from build123d import *

# Parameters (mm, degrees)
BOSS_EXTRUDE1_DEPTH        = 7.5
CUT_EXTRUDE1_DEPTH         = 1.5
F_3_1_3_1_DIAMETER_HOLE1_D = 3.1


with BuildPart() as part:
    # Sketch1 → Boss-Extrude1 (new body)
    with BuildSketch(Plane(origin=(0, 0, 0), x_dir=(1, 0, 0), z_dir=(0, 1, 0))):
        with BuildLine():
            Line((-219.119725045, 38.636719531), (-204.34760875, 36.031996866))
            ThreePointArc((-204.34760875, 36.031996866), (-207.5, 0), (-204.34760875, -36.031996866))
            Line((-204.34760875, -36.031996866), (-219.119725045, -38.636719531))
            ThreePointArc((-219.119725045, -38.636719531), (-222.5, 0), (-219.119725045, 38.636719531))
        make_face()
    extrude(amount=BOSS_EXTRUDE1_DEPTH)

    # Sketch2 → Cut-Extrude1 (cut)
    with BuildSketch(Plane(origin=(0, 7.5, 0), x_dir=(1, 0, 0), z_dir=(0, 1, 0))):
        with BuildLine():
            Line((-206.809628133, 36.46611731), (-216.657705663, 38.202599087))
            ThreePointArc((-216.657705663, 38.202599087), (-218.670303662, 24.151569236), (-219.772609758, 10))
            Line((-219.772609758, 10), (-209.761769634, 10))
            ThreePointArc((-209.761769634, 10), (-208.70564487, 23.279901188), (-206.809628133, 36.46611731))
        make_face()
        with BuildLine():
            Line((-209.761769634, -10), (-219.772609758, -10))
            ThreePointArc((-219.772609758, -10), (-218.670303662, -24.151569236), (-216.657705663, -38.202599087))
            Line((-216.657705663, -38.202599087), (-206.809628133, -36.46611731))
            ThreePointArc((-206.809628133, -36.46611731), (-208.70564487, -23.279901188), (-209.761769634, -10))
        make_face()
    extrude(amount=-CUT_EXTRUDE1_DEPTH, mode=Mode.SUBTRACT)

    # Ø3.1 (3.1) Diameter Hole1 (through all)
    with Locations(Plane(origin=(0, 0, 0), x_dir=(-1, 0, 0), z_dir=(0, -1, 0))):
        with Locations((214.18186009, -18.738484691), (214.18186009, 18.738484691)):
            Hole(F_3_1_3_1_DIAMETER_HOLE1_D / 2)


solid = part.part
Read the model definition and answer for the solid it produces. Units are mm, in the model's axes. A direction names the side the tool comes from. Round coordinates to 2 decimals unless told otherwise and drop trailing zeros. Order: outer loops, then holes, each group sorted by start corner. A loop starts at its lowest first (then second) coordinate and runs counter-clockwise, first axis right, second up.
1) For faces 5 (the face through (-208.726, 6.76, -23.095)), 6 (the face through (-208.685, 6.76, 23.465)), 7 (the face through (-215, 7, 10)), 8 (the face through (-207.5, 3.7, -0.5)), 9 (the face through (-212.75, 3.04, 19.33)), determine the directions among +Z, -Z, +X, -X, +Y, -Y from which every point of the face is accessible in a straight line to the end or side of a thin tool.
2) The part is cut by section B-B on y = 1. Write down the section's boundary in (x, z).
3) The part is cut by section C-C on x = -208.5. Write down the section's boundary in (y, z), plus the area to 3 significant figures.
4) Flat-ended cylindrical pins translate along their axes: pin 1 (2.5 mm diameter, centred on x = -214.18, z = 18.74, fed in from -Y); pin 2 (1 mm diameter, centred on y = 5, z = 12, fed in from -X); pin 3 (1.6 mm diameter, centred on x = -214, y = 7, fed in from -Z); pin 4 (2 mm diameter, centred on y = 3.5, z = -23.5, fed in from +X). Find the tip coordinate at first contact, or state that the pin passes through.
5) The mould has two halves that part along Z. Classify faces 1 (the face through (-218.692, 6.76, 23.954)), 2 (the face through (-222.5, 3.7, 0.5)), 3 (the face through (-215, 7.5, -1)), 4 (the face through (-211.63, 2.864, 37.316)): released by +Z, released by -Z, zero draft, split by the parting line, or undercut.
6) Straight lines are drawn through the part: L1, parallel to Z at x = -214, y = 3.25; L2, parallel to X at y = 3.25, z = 2; L3, parallel to Y at x = -209.5, z = -15. For each, find the intervals that lie inside material, in ascending order.
7) The part is cut by section D-D on y = 6.75. Write down the section's boundary in (x, z), plus the area to 3 significant figures.
8) The part is cut by section A-A on z = 18. Write down the section's boundary in (x, y).
Resolved:
1. face 5: -Z, +Y
1. face 6: +Z, +Y
1. face 7: +Y
1. face 8: +X, +Y, -Y
1. face 9: +Y, -Y
2. outline: (-219.12, -38.64) - (-204.35, -36.03) arc R207.5 cw to (-204.35, 36.03) - (-219.12, 38.64) arc R222.5 ccw to start; hole circle Ø3.1 at (-214.18, -18.74); hole circle Ø3.1 at (-214.18, 18.74)
3. outline: (0, -36.76) - (6, -36.76) - (6, -25.05) - (7.5, -25.05) - (7.5, 25.05) - (6, 25.05) - (6, 36.76) - (0, 36.76) - close
3. area: 516 mm2
4. pin 1: passes through
4. pin 2: stops at x = -222.2
4. pin 3: stops at z = -10
4. pin 4: stops at x = -206.05
5. face 1: undercut
5. face 2: split by the parting line
5. face 3: zero draft
5. face 4: released by +Z
6. L1: z = -37.73 to -20.28, -17.2 to 17.2, 20.28 to 37.73
6. L2: x = -222.49 to -207.49
6. L3: y = 0 to 6
7. outline: (-219.77, -10) - (-209.76, -10) arc R210 ccw to (-206.81, -36.47) - (-204.35, -36.03) arc R207.5 cw to (-204.35, 36.03) - (-206.81, 36.47) arc R210 ccw to (-209.76, 10) - (-219.77, 10) arc R220 cw to (-216.66, 38.2) - (-219.12, 38.64) arc R222.5 ccw to (-219.12, -38.64) - (-216.66, -38.2) arc R220 cw to start
7. area: 575 mm2
8. outline: (-221.77, 0) - (-215.54, 0) - (-215.54, 6) - (-219.26, 6) - (-219.26, 7.5) - (-221.77, 7.5) - close; (-212.82, 0) - (-206.72, 0) - (-206.72, 7.5) - (-209.23, 7.5) - (-209.23, 6) - (-212.82, 6) - close
